from build123d import *

# Parameters (mm, degrees)
BASE_FLANGE1_DEPTH      = 152.4
SKETCH6_W               = 50.8
SKETCH6_H               = 31.75
CUT_EXTRUDE1_DEPTH      = 348.354286896
F_3_8_CLEARANCE_HOLE1_D = 10.0838
SKETCH8_W               = 10.0838
SKETCH8_H               = 15.875
CUT_EXTRUDE2_DEPTH      = 348.354286896


# Sheet-metal steps are written as plain solids
with BuildPart() as part:
    # Sketch1 → Base-Flange1 (new, symmetric)
    with BuildSketch(Plane.XY):
        with BuildLine():
            Line((-152.4, 50.8), (-152.4, 1.5875))
            ThreePointArc((-152.4, 1.5875), (-151.935032015, 0.464967985), (-150.8125, 0))
            Line((-150.8125, 0), (150.8125, 0))
            ThreePointArc((150.8125, 0), (151.935032015, 0.464967985), (152.4, 1.5875))
            Line((152.4, 1.5875), (152.4, 50.8))
            Line((152.4, 50.8), (153.9875, 50.8))
            Line((153.9875, 50.8), (153.9875, 1.5875))
            ThreePointArc((153.9875, 1.5875), (153.05756403, -0.65756403), (150.8125, -1.5875))
            Line((150.8125, -1.5875), (-150.8125, -1.5875))
            ThreePointArc((-150.8125, -1.5875), (-153.05756403, -0.65756403), (-153.9875, 1.5875))
            Line((-153.9875, 1.5875), (-153.9875, 50.8))
            Line((-153.9875, 50.8), (-152.4, 50.8))
        make_face()
    extrude(amount=BASE_FLANGE1_DEPTH, both=True)

    # Sketch6 → Cut-Extrude1 (cut, through all)
    with BuildSketch(Plane(origin=(153.9875, 0, 0), x_dir=(0, 0, -1), z_dir=(1, 0, 0))):
        with Locations((0, 34.925)):
            Rectangle(SKETCH6_W, SKETCH6_H)
    extrude(amount=-CUT_EXTRUDE1_DEPTH, mode=Mode.SUBTRACT)

    # 3/8 Clearance Hole1 (through all)
    with Locations(Plane(origin=(153.9875, 34.925, 123.825), x_dir=(0, 0, 1), z_dir=(1, 0, 0))):
        with Locations((0, 0), (-247.65, 0)):
            Hole(F_3_8_CLEARANCE_HOLE1_D / 2)

    # Sketch8 → Cut-Extrude2 (cut, through all)
    with BuildSketch(Plane(origin=(153.9875, 0, 0), x_dir=(0, 0, -1), z_dir=(1, 0, 0))):
        with Locations((-123.825, 42.8625)):
            Rectangle(SKETCH8_W, SKETCH8_H)
        with Locations((123.825, 42.8625)):
            Rectangle(SKETCH8_W, SKETCH8_H)
    extrude(amount=-CUT_EXTRUDE2_DEPTH, mode=Mode.SUBTRACT)


solid = part.part
Work out the finished part from the listing and answer in its coordinate system (mm). A direction names the side the tool comes from. Give positions to 0.01 mm unless a question says otherwise; leave off trailing zeros. Loops run counter-clockwise (first coordinate to the right, second up) from the corner with the lowest first, then second, coordinate; pieces in that order, holes last. Notation, with made-up numbers: (-39.75, -12.75) -> (17.25, -12.75) arc R19 cw to (17.25, 5.25) -> close; hole circle Ø5 at (63, 33.25). An arc over 180 degrees is marked (long way). Use a Markdown table: item, result. Add a question column.
1) The part is cut by section D-D, the plane x = -79. Determine the outline of the cut face in (y, z), plus the area to 3 significant figures.
2) Which of the six approach directions +Z, -Z, +X, -X, +Y, -Y give full straight-line access (tool end or side, diameter ignored) to faces 4 (the flat face through (-153.988, 15, 2)), 5 (the flat face through (-152.4, 16, 2))?
3) Consider line 1 along X through (y, z) = (27, 81); line 2 along Y through (x, z) = (73.5, 60). Determine where each line is inside the solid, lowest interval first.
4) Each of these flat-tipped pins is pushed along its axis until it touches: P1, Ø5, axis at x = -24.5, z = -56, coming from the +Y side; P2, Ø0.5, axis at x = 153.5, z = -1, coming from the +Y side. Where does it stop, or does it pass through?
5) The part is cut by section A-A, the plane y = 43. Count the separate pieces of the cut face and the enclosed holes in it, plus the area to 3 significant figures.
6) The part is cut by section B-B, the plane y = 14. Determine the outline of the cut face in (x, z), plus the area to 3 significant figures.
7) For a pull along X with two mould halves and no side action, classify faces 1 (the flat face through (-2, 0, 2)), 2 (the flat face through (153.988, 16, 2)), 3 (the flat face through (0.7, -0.5, -152.4)) as +X half, -X half, draft (parallel to the pull), parting line (faces both ways), or undercut.
Reported:
| question | item | result |
|---|---|---|
| 1 | outline | (-1.59, -152.4) -> (0, -152.4) -> (0, 152.4) -> (-1.59, 152.4) -> close |
| 1 | area | 484 mm^2 |
| 2 | face 4 | +Z, -Z, -X, +Y, -Y |
| 2 | face 5 | +Z, -Z, +Y |
| 3 | line 1 | x = -153.99 to -152.4, 152.4 to 153.99 |
| 3 | line 2 | y = -1.59 to 0 |
| 4 | P1 | stops at y = 0 |
| 4 | P2 | stops at y = 19.05 |
| 5 | separate pieces | 8 |
| 5 | enclosed holes | 0 |
| 5 | area | 742 mm^2 |
| 6 | outline | (-153.99, -152.4) -> (-152.4, -152.4) -> (-152.4, 152.4) -> (-153.99, 152.4) -> close; (152.4, -152.4) -> (153.99, -152.4) -> (153.99, 152.4) -> (152.4, 152.4) -> close |
| 6 | area | 968 mm^2 |
| 7 | face 1 | undercut |
| 7 | face 2 | +X half |
| 7 | face 3 | draft |
